Work out the finished part from the listing and answer in its coordinate system (mm). Face numbers are marked on the shaded views. A direction names the side the tool comes from. Coordinates: 2 decimals unless noted, no trailing zeros. Loops run counter-clockwise (first coordinate to the right, second up) from the corner with the lowest first, then second, coordinate; pieces in that order, holes last. Notation, with made-up numbers: (-2.75, 1) -> (29.25, 1) arc R19 ccw to (29.25, 34) -> close; hole circle Ø8 at (-15.5, -26). An arc over 180 degrees is marked (long way). Answer as CSV lines item,"result".
```python
from build123d import *

# Parameters (mm, degrees)
SKETCH1_W            = 20
SKETCH1_H            = 47.5
BOSS_EXTRUDE1_DEPTH  = 2.5
SKETCH2_R            = 20
BOSS_EXTRUDE2_DEPTH  = 5
SKETCH3_R            = 15
BOSS_EXTRUDE3_DEPTH  = 5
SKETCH4_R            = 20
BOSS_EXTRUDE4_DEPTH  = 5
SKETCH5_R            = 15
BOSS_EXTRUDE5_DEPTH  = 5
SKETCH6_R            = 20
BOSS_EXTRUDE6_DEPTH  = 5
BOSS_EXTRUDE7_DEPTH  = 2.5
SKETCH8_W            = 30
SKETCH8_H            = 20
BOSS_EXTRUDE8_DEPTH  = 2.5
SKETCH10_W           = 20
SKETCH10_H           = 2.5
BOSS_EXTRUDE9_DEPTH  = 25
SKETCH11_R           = 15
BOSS_EXTRUDE10_DEPTH = 2.5
SKETCH12_R           = 15
BOSS_EXTRUDE11_DEPTH = 2.5
FILLET1_R            = 2.5
FILLET2_R            = 2.5


with BuildPart() as part:
    # Sketch1 → Boss-Extrude1 (new body)
    with BuildSketch(Plane(origin=(0, 0, 0), x_dir=(0, 0, -1), z_dir=(1, 0, 0))):
        with Locations((0, -1.25)):
            Rectangle(SKETCH1_W, SKETCH1_H)
    extrude(amount=BOSS_EXTRUDE1_DEPTH)

    # Sketch2 → Boss-Extrude2 (add)
    with BuildSketch(Plane(origin=(2.5, 0, 0), x_dir=(0, 0, -1), z_dir=(1, 0, 0))):
        Circle(SKETCH2_R)
    extrude(amount=BOSS_EXTRUDE2_DEPTH)

    # Sketch3 → Boss-Extrude3 (add)
    with BuildSketch(Plane(origin=(7.5, 0, 0), x_dir=(0, 0, -1), z_dir=(1, 0, 0))):
        Circle(SKETCH3_R)
    extrude(amount=BOSS_EXTRUDE3_DEPTH)

    # Sketch4 → Boss-Extrude4 (add)
    with BuildSketch(Plane(origin=(12.5, 0, 0), x_dir=(0, 0, -1), z_dir=(1, 0, 0))):
        Circle(SKETCH4_R)
    extrude(amount=BOSS_EXTRUDE4_DEPTH)

    # Sketch5 → Boss-Extrude5 (add)
    with BuildSketch(Plane(origin=(17.5, 0, 0), x_dir=(0, 0, -1), z_dir=(1, 0, 0))):
        Circle(SKETCH5_R)
    extrude(amount=BOSS_EXTRUDE5_DEPTH)

    # Sketch6 → Boss-Extrude6 (add)
    with BuildSketch(Plane(origin=(22.5, 0, 0), x_dir=(0, 0, -1), z_dir=(1, 0, 0))):
        Circle(SKETCH6_R)
    extrude(amount=BOSS_EXTRUDE6_DEPTH)

    # Sketch7 → Boss-Extrude7 (add)
    with BuildSketch(Plane(origin=(27.5, 0, 0), x_dir=(0, 0, -1), z_dir=(1, 0, 0))):
        Polygon((-10, -22.5), (-10, -25), (10, -25), (10, -22.5), (10, 22.5), (-10, 22.5), align=None)
    extrude(amount=BOSS_EXTRUDE7_DEPTH)

    # Sketch8 → Boss-Extrude8 (add)
    with BuildSketch(Plane(origin=(0, 22.5, 0), x_dir=(1, 0, 0), z_dir=(0, 1, 0))):
        with Locations((15, 0)):
            Rectangle(SKETCH8_W, SKETCH8_H)
    extrude(amount=BOSS_EXTRUDE8_DEPTH)

    # Sketch10 → Boss-Extrude9 (add)
    with BuildSketch(Plane(origin=(2.5, 0, 0), x_dir=(0, 0, -1), z_dir=(1, 0, 0))):
        with Locations((0, -23.75)):
            Rectangle(SKETCH10_W, SKETCH10_H)
    extrude(amount=BOSS_EXTRUDE9_DEPTH)

    # Sketch11 → Boss-Extrude10 (add)
    with BuildSketch(Plane(origin=(30, 0, 0), x_dir=(0, 0, -1), z_dir=(1, 0, 0))):
        Circle(SKETCH11_R)
    extrude(amount=-BOSS_EXTRUDE10_DEPTH)

    # Sketch12 → Boss-Extrude11 (add)
    with BuildSketch(Plane.ZY):
        Circle(SKETCH12_R)
    extrude(amount=-BOSS_EXTRUDE11_DEPTH)

    # Fillet1
    fillet1_edges = [part.edges().sort_by_distance(p)[0] for p in [
        (0, 25, 0),
        (30, 25, 0),
    ]]
    fillet(fillet1_edges, radius=FILLET1_R)

    # Fillet2
    fillet2_edges = [part.edges().sort_by_distance(p)[0] for p in [
        (30, -25, 0),
        (0, -25, 0),
    ]]
    fillet(fillet2_edges, radius=FILLET2_R)


solid = part.part
```
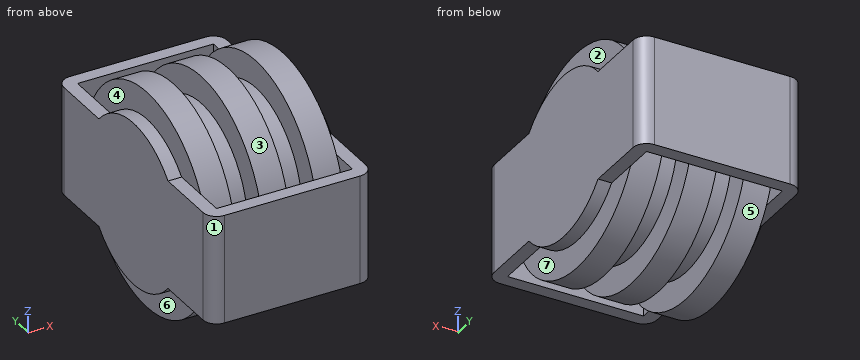
(1) A cutting plane is placed at C-C, the plane y = 0. Write down the section's boundary in (x, z).
Computed values:
outline,"(0, -15) -> (2.5, -15) -> (2.5, -20) -> (7.5, -20) -> (7.5, -15) -> (12.5, -15) -> (12.5, -20) -> (17.5, -20) -> (17.5, -15) -> (22.5, -15) -> (22.5, -20) -> (27.5, -20) -> (27.5, -15) -> (30, -15) -> (30, 15) -> (27.5, 15) -> (27.5, 20) -> (22.5, 20) -> (22.5, 15) -> (17.5, 15) -> (17.5, 20) -> (12.5, 20) -> (12.5, 15) -> (7.5, 15) -> (7.5, 20) -> (2.5, 20) -> (2.5, 15) -> (0, 15) -> close"
(2) For a pull along Y with two mould halves and no side action, classify the marked faces 1, 2 and 3 as pulls with the +Y half, pulls with the -Y half, needs draft (parallel to the pull), parting line crosses it, or undercut.
Computed values:
face 1,"pulls with the -Y half"
face 2,"needs draft"
face 3,"undercut"
(3) Flat-ended cylindrical pins translate along their axes: pin 1 Ø6 at (x, y) = (7, 10) entering from -Z (3 decimals); pin 2 Ø1 at (x, y) = (5, -15.5) entering from -Z; pin 3 Ø11 at (x, y) = (13.5, 17.5) entering from -Z. Find the tip coordinate at first contact, or state that the pin passes through.
Computed values:
pin 1,"z = -18.735"
pin 2,"z = -13.23"
pin 3,"z = -16"
(4) Consider line 1 along X through (y, z) = (-18.5, -4); line 2 along Y through (x, z) = (20, -5); line 3 along X through (y, z) = (-21.5, -9). Determine where each line is inside the solid, lowest interval first.
Computed values:
line 1,"0 to 7.5, 12.5 to 17.5, 22.5 to 30"
line 2,"-25 to -22.5, -14.14 to 14.14, 22.5 to 25"
line 3,"0 to 2.5, 27.5 to 30"
(5) A cutting plane is placed at B-B, the plane z = 0. Count the separate pieces of the cut face and the enclosed holes in it, and give its area (3 significant figures).
Computed values:
separate pieces,"1"
enclosed holes,"2"
area,"1,270 mm2"
(6) Which of the six approach directions +Z, -Z, +X, -X, +Y, -Y give full straight-line access (tool end or side, diameter ignored) to the marked faces 4, 5, 6 and 7?
Computed values:
face 4,"+Z, -X"
face 5,"none"
face 6,"-Z, -X"
face 7,"-Z, +X"
(7) A cutting plane is placed at A-A, the plane x = 26.5. Write down the section's boundary in (y, z), and give its area (3 significant figures).
Computed values:
outline,"(-25, -10) -> (-22.5, -10) -> (-22.5, 10) -> (-25, 10) -> close; circle Ø40 at (0, 0); (22.5, -10) -> (25, -10) -> (25, 10) -> (22.5, 10) -> close"
area,"1,360 mm2"
